The drawing under review shows one solid part. Ordinate dimensions are in mm from its lowest x, y, z. Round coordinates to 2 decimals unless told otherwise and drop trailing zeros. Order: outer loops, then holes, each group sorted by start corner. A loop starts at its lowest first (then second) coordinate and runs counter-clockwise, first axis right, second up.
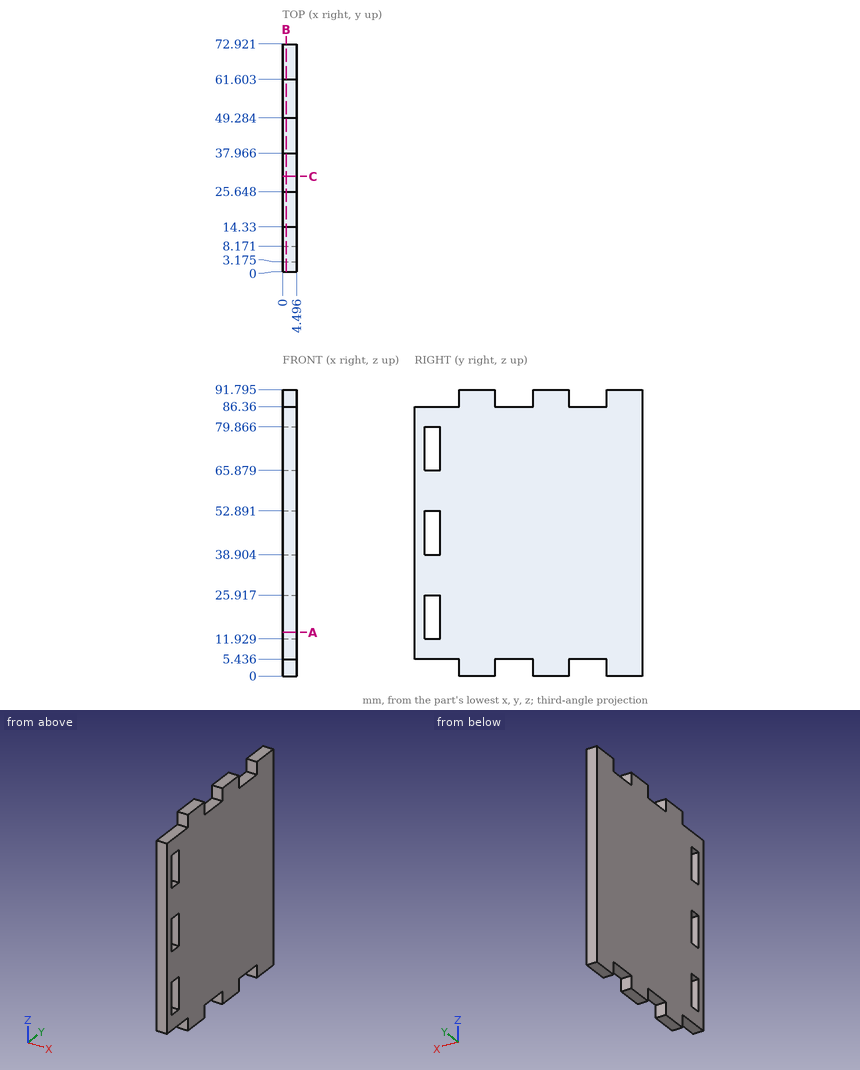
Q1. Take a section at B-B, the plane x = 1.1. Count the separate pieces of the cut face and the enclosed holes in it, plus the area to 3 significant figures.
Q2. Take a section at A-A, the plane z = 14. State the section outline as (x, y) points (1 decimal).
Q3. Wall thickness on line 1 (Z direction, x = 0.85, y = 4) (1 decimal); line 2 (Y direction, x = 0.8, z = 24) (1 decimal); line 3 (Z direction, x = 2.6, y = 61.5) (1 decimal): over which ranges is each line inside the solid? List them lowest first.
Q4. Clearance check with flat-ended pins moving along their axes: pin 1 (2 mm diameter, centred on x = 1.5, z = 45, fed in from -Y); pin 2 (2 mm diameter, centred on x = 3, y = 29.5, fed in from +Z). State where each tip first meets the part, or that it passes through.
Q5. Take a section at C-C, the plane y = 30.5. State the section outline as (x, z) points (1 decimal), plus the area to 3 significant figures.
Working result:
1. separate pieces: 1
1. enclosed holes: 3
1. area: 6,060 mm2
2. outline: (0, 0) - (4.5, 0) - (4.5, 3.2) - (0, 3.2) - close; (0, 8.2) - (4.5, 8.2) - (4.5, 72.9) - (0, 72.9) - close
3. line 1: z = 5.4 to 11.9, 25.9 to 38.9, 52.9 to 65.9, 79.9 to 86.4
3. line 2: y = 0 to 3.2, 8.2 to 72.9
3. line 3: z = 5.4 to 86.4
4. pin 1: stops at y = 0
4. pin 2: stops at z = 86.36
5. outline: (0, 5.4) - (4.5, 5.4) - (4.5, 86.4) - (0, 86.4) - close
5. area: 364 mm2
